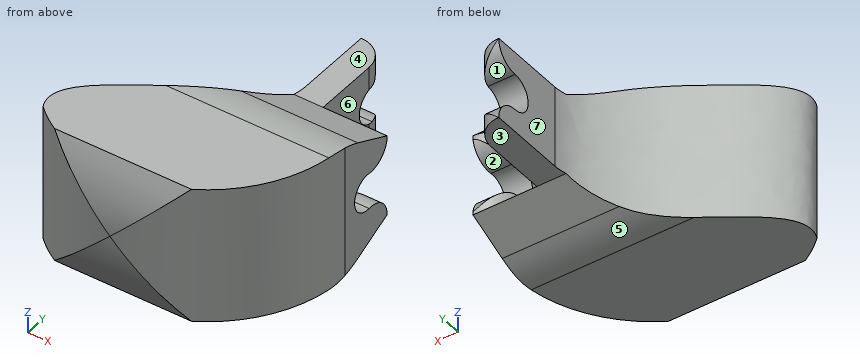
```python
from build123d import *

# Parameters (mm, degrees)
SKETCH1_R                = 2
SKETCH1_R_2              = 2.6
BOSS_EXTRUDE1_DEPTH      = 9
FILLET1_R                = 4
SKETCH3_W                = 1
SKETCH3_H                = 25
CUT_EXTRUDE2_DEPTH       = 131.694299799
CUT_EXTRUDE3_DEPTH       = 132.837020597
BOSS_EXTRUDE2_DEPTH      = 3
BOSS_EXTRUDE4_DEPTH      = 5
CUT_EXTRUDE4_DEPTH       = 2
FILLET2_R                = 20
FILLET3_R                = 4
BOSS_EXTRUDE5_DEPTH      = 12
BOSS_EXTRUDE5_DEPTH_BACK = 3
CUT_EXTRUDE5_DEPTH       = 134.026557597
CUT_EXTRUDE5_DEPTH_BACK  = 134.026557597


with BuildPart() as part:
    # Sketch1 → Boss-Extrude1 (new body)
    with BuildSketch(Plane.XY):
        Polygon((0, 0), (-10, 0), (-10, 30), (-20, 90), (-20, 130), (-10, 130), (-10, 90), (0, 30), align=None)
        with Locations((-15, 100)):
            Circle(SKETCH1_R, mode=Mode.SUBTRACT)
        with Locations((-15, 125)):
            Circle(SKETCH1_R_2, mode=Mode.SUBTRACT)
    extrude(amount=BOSS_EXTRUDE1_DEPTH)

    # Fillet1
    fillet1_edges = [part.edges().sort_by_distance(p)[0] for p in [
        (0, 0, 4.5),
        (-10, 0, 4.5),
    ]]
    fillet(fillet1_edges, radius=FILLET1_R)

    # Sketch3 → Cut-Extrude2 (cut, through all)
    with BuildSketch(Plane.ZY.offset(10)):
        with Locations((0.5, 117.5)):
            Rectangle(SKETCH3_W, SKETCH3_H)
    extrude(amount=CUT_EXTRUDE2_DEPTH, mode=Mode.SUBTRACT)

    # Sketch5 → Cut-Extrude3 (cut, through all)
    with BuildSketch(Plane.XY.offset(9)):
        with BuildLine():
            Line((-10, 4), (-10, 24))
            ThreePointArc((-10, 24), (-7.878679656, 23.121320344), (-7, 21))
            Line((-7, 21), (-7, 6))
            ThreePointArc((-7, 6), (-5, 4), (-3, 6))
            Line((-3, 6), (-3, 10.96659189))
            ThreePointArc((-3, 10.96659189), (-2.121320344, 13.087912234), (0, 13.96659189))
            Line((0, 13.96659189), (0, 4))
            ThreePointArc((0, 4), (-1.171572875, 1.171572875), (-4, 0))
            Line((-4, 0), (-6, 0))
            ThreePointArc((-6, 0), (-8.828427125, 1.171572875), (-10, 4))
        make_face()
    extrude(amount=-CUT_EXTRUDE3_DEPTH, mode=Mode.SUBTRACT)

    # Boss-Extrude2: read off the stored shape, not the designer's step
    # Boss-Extrude2 outline → Boss-Extrude2 (add)
    with BuildSketch(Plane.ZY):
        with BuildLine():
            Line((9, 13.96659189), (9, 30))
            Line((9, 30), (0, 30))
            Line((0, 30), (0, 13.96659189))
            Line((0, 13.96659189), (0.423395215, 13.96659189))
            ThreePointArc((0.423395215, 13.96659189), (2.009052541, 13.008624555), (2.499994655, 11.222291324))
            ThreePointArc((2.499994655, 11.222291324), (4.487608253, 9.000047793), (6.47522185, 11.222291324))
            ThreePointArc((6.47522185, 11.222291324), (6.966163965, 13.008624555), (8.551821291, 13.96659189))
            Line((8.551821291, 13.96659189), (9, 13.96659189))
        make_face()
    extrude(amount=BOSS_EXTRUDE2_DEPTH)

    # Sketch8 → Boss-Extrude4 (add)
    with BuildSketch(Plane.ZY.offset(10)):
        with BuildLine():
            Line((2.5, 21.5), (6.5, 21.5))
            ThreePointArc((6.5, 21.5), (4.5, 19.5), (2.5, 21.5))
        make_face()
        with BuildLine():
            ThreePointArc((0, 24), (1.767766953, 23.267766953), (2.5, 21.5))
            Line((2.5, 21.5), (6.5, 21.5))
            ThreePointArc((6.5, 21.5), (7.232233047, 23.267766953), (9, 24))
            Line((9, 24), (0, 24))
        make_face()
    extrude(amount=-BOSS_EXTRUDE4_DEPTH)

    # Sketch9 → Cut-Extrude4 (cut)
    with BuildSketch(Plane(origin=(4.931969619, 0.408182285, 0), x_dir=(0, 0, -1), z_dir=(0.9863939238321437, 0.16439898730535749, 0))):
        with BuildLine():
            Line((-7, 37), (-7, 85.827625303))
            ThreePointArc((-7, 85.827625303), (-4.5, 88.327625303), (-2, 85.827625303))
            Line((-2, 85.827625303), (-2, 37))
            ThreePointArc((-2, 37), (-4.5, 34.5), (-7, 37))
        make_face()
    cut_extrude4 = extrude(amount=-CUT_EXTRUDE4_DEPTH, mode=Mode.SUBTRACT)

    # Mirror1: Cut-Extrude4 across plane
    add(cut_extrude4.mirror(Plane(origin=(0, 0, 0), x_dir=(0, 0, 1), z_dir=(0.9863939238321437, 0.16439898730535743, 0))), mode=Mode.SUBTRACT)

    # Fillet2
    fillet2_edges = [part.edges().sort_by_distance(p)[0] for p in [
        (-10, 30, 4.5),
        (-20, 90, 4.5),
        (-10, 90, 4.5),
        (0, 30, 4.5),
    ]]
    fillet(fillet2_edges, radius=FILLET2_R)

    # Fillet3
    fillet3_edges = [part.edges().sort_by_distance(p)[0] for p in [
        (-20, 130, 5),
        (-10, 130, 5),
    ]]
    fillet(fillet3_edges, radius=FILLET3_R)


with BuildPart() as body_2:
    # Sketch1<5> → Boss-Extrude5 (new, two sides: drawn at the far end of the back side and taken through both)
    with BuildSketch(Plane.XY.offset(-BOSS_EXTRUDE5_DEPTH_BACK)):
        with BuildLine():
            ThreePointArc((-25.154949118, -3.539792045), (-8.971908958, -6.235432952), (0, 7.5))
            Line((0, 7.5), (0, 27.350317066))
            Line((0, 27.350317066), (-10, 27.350317066))
            Line((-10, 27.350317066), (-10, 15.414300315))
            add(Edge.make_bspline(
                [(-10, 15.414300315), (-10.3332076, 5.995566791), (-28.355100317, 2.568910038), (-25.154949118, -3.539792045)],
                knots=[0, 0, 0, 0, 0.764316477, 0.764316477, 0.764316477, 0.764316477], degree=3))
        make_face()
    extrude(amount=BOSS_EXTRUDE5_DEPTH + BOSS_EXTRUDE5_DEPTH_BACK)

    # Sketch10 → Cut-Extrude5 (cut, two sides: drawn at the far end of the back side and taken through both)
    with BuildSketch(Plane(origin=(0, 0, 0), x_dir=(0, 0, -1), z_dir=(1, 0, 0)).offset(-CUT_EXTRUDE5_DEPTH_BACK)):
        with BuildLine():
            Line((-9, 13.96659189), (-9, 28.344749394))
            Line((-9, 28.344749394), (-14.199341922, 29.234870168))
            Line((-14.199341922, 29.234870168), (-18.34923463, 5.372987094))
            Line((-18.34923463, 5.372987094), (-14.775715909, -10.880759347))
            Line((-14.775715909, -10.880759347), (12.313861494, -10.073835765))
            Line((12.313861494, -10.073835765), (10.584739532, 28.344749394))
            Line((10.584739532, 28.344749394), (0, 28.344749394))
            Line((0, 28.344749394), (0, 13.96659189))
            Line((0, 13.96659189), (2.071346392, 9.501741297))
            ThreePointArc((2.071346392, 9.501741297), (2.765077161, 7.448160424), (3, 5.29333606))
            Line((3, 5.29333606), (3, -5.490381057))
            ThreePointArc((3, -5.490381057), (-4.5, -7.5), (-12, -5.490381057))
            Line((-12, -5.490381057), (-12, 5.29333606))
            ThreePointArc((-12, 5.29333606), (-11.765077161, 7.448160424), (-11.071346392, 9.501741297))
            Line((-11.071346392, 9.501741297), (-9, 13.96659189))
        make_face()
    extrude(amount=CUT_EXTRUDE5_DEPTH + CUT_EXTRUDE5_DEPTH_BACK, mode=Mode.SUBTRACT)

    # Combine1: cut part
    add(part.part, mode=Mode.SUBTRACT)


solid = body_2.part
```
Work out the finished part from the listing and answer in its coordinate system (mm). Face numbers are marked on the shaded views. A direction names the side the tool comes from. Give positions to 0.01 mm unless a question says otherwise; leave off trailing zeros. Write each loop counter-clockwise with the first axis right and the second up, starting at its lowest first coordinate (ties: lowest second). Pieces come first, ordered by that corner, then holes. Notation, with made-up numbers: (85, 5.25) -> (109, 5.25) arc R20 cw to (109, 19.25) -> close; hole circle Ø9 at (-4, -28). An arc over 180 degrees is marked (long way). Write item = value, one per line.
Q1. A tool of negligible diameter and unlimited length cuts with its end or side. For the marked faces 1, 2, 3 and 4, from which of +Z, -Z, +X, -X, +Y, -Y can it reach the whole face along a straight path? Write none if from no direction.
Computed values:
face_1 = +X, -X, +Y
face_2 = +X
face_3 = -Z, +X, -X, +Y
face_4 = +Z, +X, -X, +Y
Q2. Consider line 1 along X through (y, z) = (18.5, 6.5); line 2 along X through (y, z) = (6.5, 5); line 3 along X through (y, z) = (7.5, -1). Determine where each line is inside the solid, lowest interval first.
Computed values:
line_1 = -10 to -7
line_2 = -16.31 to -7, -3 to -0.03
line_3 = -15 to 0
Q3. Section B-B on y = -4.5 is taken. Determine the outline of the cut face in (x, z), and give its area (3 significant figures).
Computed values:
outline = (-24, -3) -> (-6, -3) -> (-6, 12) -> (-24, 12) -> close
area = 270 mm^2
Q4. For a pull along X with two mould halves and no side action, classify the marked faces 5, 6 and 7 as pulls with the +X half, pulls with the -X half, needs draft (parallel to the pull), parting line crosses it, or undercut.
Computed values:
face_5 = needs draft
face_6 = undercut
face_7 = pulls with the -X half
Q5. Section A-A on x = -5 is taken. Determine the outline of the cut face in (y, z), and give its area (3 significant figures).
Computed values:
outline = (-3.68, -3) -> (5.29, -3) arc R10 ccw to (9.5, -2.07) -> (13.97, 0) -> (4, 0) -> (4, 9) -> (13.97, 9) -> (9.5, 11.07) arc R10 ccw to (5.29, 12) -> (-3.68, 12) -> close
area = 155 mm^2
Q6. Flat-ended cylindrical pins translate along their axes: pin 1 Ø2 at (x, z) = (-15.5, 3) entering from -Y; pin 2 Ø8 at (y, z) = (6.5, 4.5) entering from +X; pin 3 Ø2.5 at (x, y) = (-8, 17) entering from +Z; pin 4 Ø4 at (x, y) = (-4.5, 18) entering from -Z. Find the tip coordinate at first contact, or state that the pin passes through.
Computed values:
pin_1 = -7.49
pin_2 = 0
pin_3 = 9
pin_4 = through
